The figure shows three views and two pictorial views of one solid part (mm, origin at its lowest corner). Answer the questions. A direction names the side the tool comes from. Coordinates: 2 decimals unless noted, no trailing zeros. Order: outer loops, then holes, each group sorted by start corner. A loop starts at its lowest first (then second) coordinate and runs counter-clockwise, first axis right, second up. Notation, with made-up numbers: (67, 49) -> (84, 49) arc R12 cw to (84, 69) -> close; hole circle Ø2 at (16.5, 38). An arc over 180 degrees is marked (long way). Return JSON: item names as keys, results as strings.
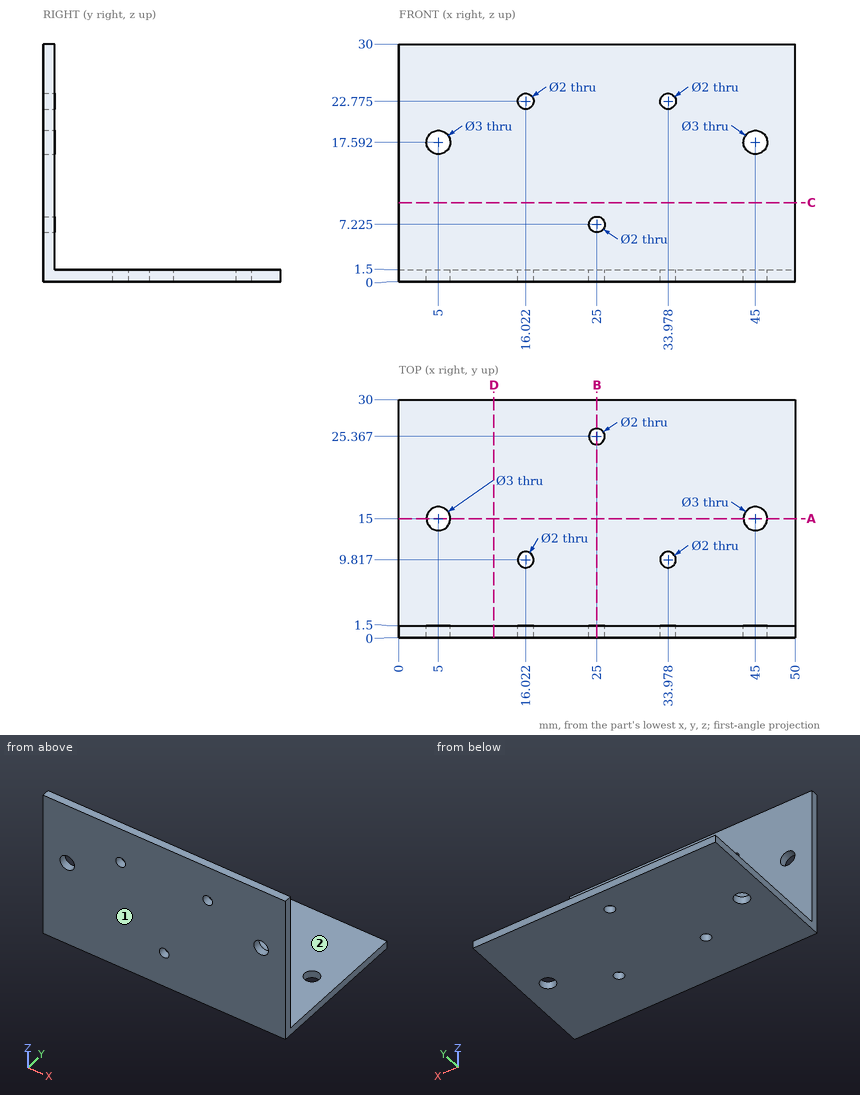
Item 1: The part is cut by section A-A on y = 15. Determine the outline of the cut face in (x, z).
Answer list:
{"outline": "(0, 0) -> (3.5, 0) -> (3.5, 1.5) -> (0, 1.5) -> close; (6.5, 0) -> (43.5, 0) -> (43.5, 1.5) -> (6.5, 1.5) -> close; (46.5, 0) -> (50, 0) -> (50, 1.5) -> (46.5, 1.5) -> close"}
Item 2: The part is cut by section D-D on x = 12. Determine the outline of the cut face in (y, z).
Answer list:
{"outline": "(0, 0) -> (30, 0) -> (30, 1.5) -> (1.5, 1.5) -> (1.5, 30) -> (0, 30) -> close"}
Item 3: Flat-ended cylindrical pins translate along their axes: pin 1 (3 mm diameter, centred on x = 16.02, z = 22.78, fed in from +Y); pin 2 (4 mm diameter, centred on x = 20, y = 9.5, fed in from +Z). Find the tip coordinate at first contact, or state that the pin passes through.
Answer list:
{"pin 1": "y = 1.5", "pin 2": "z = 1.5"}
Item 4: Which of the six approach directions +Z, -Z, +X, -X, +Y, -Y give full straight-line access (tool end or side, diameter ignored) to the marked faces 1 and 2?
Answer list:
{"face 1": "+Z, -Z, +X, -X, -Y", "face 2": "+Z, +X, -X, +Y"}
Item 5: The part is cut by section B-B on x = 25. Determine the outline of the cut face in (y, z) (1 decimal).
Answer list:
{"outline": "(0, 0) -> (24.4, 0) -> (24.4, 1.5) -> (1.5, 1.5) -> (1.5, 6.2) -> (0, 6.2) -> close; (0, 8.2) -> (1.5, 8.2) -> (1.5, 30) -> (0, 30) -> close; (26.4, 0) -> (30, 0) -> (30, 1.5) -> (26.4, 1.5) -> close"}
Item 6: Find the intervals of material crossed by probe 1 along X at (y, z) = (15, 0.9); probe 2 along Y at (x, z) = (25, 0.45); probe 3 along Y at (x, z) = (45, 0.95), in increasing order.
Answer list:
{"probe 1": "0 to 3.5, 6.5 to 43.5, 46.5 to 50", "probe 2": "0 to 24.37, 26.37 to 30", "probe 3": "0 to 13.5, 16.5 to 30"}
Item 7: The part is cut by section C-C on z = 10. Determine the outline of the cut face in (x, y).
Answer list:
{"outline": "(0, 0) -> (50, 0) -> (50, 1.5) -> (0, 1.5) -> close"}
